Read the model definition and answer for the solid it produces. Units are mm, in the model's axes. A direction names the side the tool comes from. Coordinates: 2 decimals unless noted, no trailing zeros. Loops run counter-clockwise (first coordinate to the right, second up) from the corner with the lowest first, then second, coordinate; pieces in that order, holes last. Notation, with made-up numbers: (78, -21.5) - (102, -21.5) arc R8 cw to (102, -15.5) - close; hole circle Ø8 at (32, 8). An arc over 180 degrees is marked (long way). Use one line per item in the form item = value.
from build123d import *

# Parameters (mm, degrees)
SKETCH1_W           = 86
SKETCH1_H           = 55
BOSS_EXTRUDE1_DEPTH = 3.3
BOSS_EXTRUDE2_DEPTH = 17.7
SKETCH3_W           = 58
SKETCH3_H           = 12
BOSS_EXTRUDE3_DEPTH = 9.5


with BuildPart() as part:
    # Sketch1 → Boss-Extrude1 (new body)
    with BuildSketch(Plane(origin=(0, 0, 0), x_dir=(1, 0, 0), z_dir=(0, 1, 0))):
        Rectangle(SKETCH1_W, SKETCH1_H)
    extrude(amount=BOSS_EXTRUDE1_DEPTH)

    # Sketch2 → Boss-Extrude2 (add)
    with BuildSketch(Plane(origin=(0, 3.3, 0), x_dir=(1, 0, 0), z_dir=(0, 1, 0))):
        Polygon((43, 27.5), (-43, 27.5), (-43, 25), (-36.5, 25), (-36.5, -27.5), (36.5, -27.5), (36.5, 25), (43, 25), align=None)
    extrude(amount=BOSS_EXTRUDE2_DEPTH)

    # Sketch3 → Boss-Extrude3 (add)
    with BuildSketch(Plane.XY.offset(27.5)):
        with Locations((-2.5, 11)):
            Rectangle(SKETCH3_W, SKETCH3_H)
    extrude(amount=BOSS_EXTRUDE3_DEPTH)


solid = part.part
Item 1: Find the intervals of material crossed by L1, parallel to Z at x = 25, y = 19.5; L2, parallel to X at y = 19.5, z = -24; L3, parallel to X at y = 12.25, z = 34, in increasing order.
Results below:
L1 = -27.5 to 27.5
L2 = -36.5 to 36.5
L3 = -31.5 to 26.5
Item 2: Which of the six approach directions +Z, -Z, +X, -X, +Y, -Y give full straight-line access (tool end or side, diameter ignored) to faces 1 (the flat face through (-3, 17, 32)), 2 (the flat face through (-40, 3.3, 1)), 3 (the flat face through (26.5, 11, 32))?
Results below:
face_1 = +Z, +X, -X, +Y
face_2 = +Z, -X, +Y
face_3 = +Z, +X, +Y, -Y
Item 3: The part is cut by section A-A on y = 18.75. Give the vertices of the cut face in (x, z), plus the area to 3 significant figures.
Results below:
outline = (-43, -27.5) - (43, -27.5) - (43, -25) - (36.5, -25) - (36.5, 27.5) - (-36.5, 27.5) - (-36.5, -25) - (-43, -25) - close
area = 4,050 mm²
Item 4: The part is cut by section C-C on x = 35.5. Give the vertices of the cut face in (y, z), plus the area to 4 significant figures.
Results below:
outline = (0, -27.5) - (21, -27.5) - (21, 27.5) - (0, 27.5) - close
area = 1,155 mm²
Item 5: The part is cut by section B-B on z = 9.5. Give the vertices of the cut face in (x, y).
Results below:
outline = (-43, 0) - (43, 0) - (43, 3.3) - (36.5, 3.3) - (36.5, 21) - (-36.5, 21) - (-36.5, 3.3) - (-43, 3.3) - close
Item 6: Each of these flat-tipped pins is pushed along its axis until it touches: P1, Ø6, axis at y = 14, z = 7.5, coming from the -X side; P2, Ø6, axis at x = 31, z = 13.5, coming from the -Y side; P3, Ø3, axis at x = 41.5, z = -2.5, coming from the +Y side; P4, Ø3, axis at x = 40, y = 16, coming from the +Z side. Where does it stop, or does it pass through?
Results below:
P1 = -36.5
P2 = 0
P3 = 3.3
P4 = -25
Item 7: The part is cut by section D-D on y = 11.5. Give the vertices of the cut face in (x, z).
Results below:
outline = (-43, -27.5) - (43, -27.5) - (43, -25) - (36.5, -25) - (36.5, 27.5) - (26.5, 27.5) - (26.5, 37) - (-31.5, 37) - (-31.5, 27.5) - (-36.5, 27.5) - (-36.5, -25) - (-43, -25) - close
